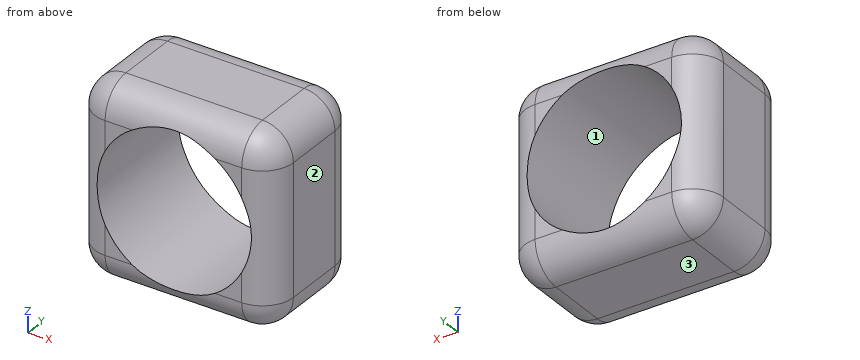
Autodesk Inventor part; units mm, degrees
ref_plane "YZ Plane" through (0, 0, 0) normal (1, 0, 0) x (0, 1, 0)
ref_plane "XZ Plane" through (0, 0, 0) normal (0, 1, 0) x (-1, 0, 0)
ref_plane "XY Plane" through (0, 0, 0) normal (0, 0, 1) x (1, 0, 0)
sketch "Sketch1" plane through (0, 0, 0) normal (0, 1, 0) x (-1, 0, 0)
  circle A0 centre (0, 0) radius 5
  line L0 (6.4276, 6.2219) -> (-6.4276, 6.2219)
  line L1 (-6.4276, 6.2219) -> (-6.4276, -6.2219)
  line L2 (-6.4276, -6.2219) -> (6.4276, -6.2219)
  line L3 (6.4276, -6.2219) -> (6.4276, 6.2219)
  line L4 (6.4276, 6.2219) -> (-6.4276, -6.2219) construction
  line L5 (-6.4276, 6.2219) -> (6.4276, -6.2219) construction
  dimension "d0" = 10
extrude "Extrusion1" add sketch "Sketch1" along normal blind 8
fillet "Fillet1" radius 2 12 edges at (6.4276, 8, 0) (0, 8, -6.2219) (0, 8, 6.2219) (-6.4276, 8, 0) (-6.4276, 0, 0) (0, 0, 6.2219) (6.4276, 0, 0) (0, 0, -6.2219) (-6.4276, 4, -6.2219) (6.4276, 4, 6.2219) (6.4276, 4, -6.2219) (-6.4276, 4, 6.2219)
thread "Thread1"
properties part number "benzcadnut"
The model under review builds one solid part; all positions refer to its coordinate system, in mm. Face numbers are marked on the shaded views. Round coordinates to 2 decimals unless told otherwise and drop trailing zeros. Order: outer loops, then holes, each group sorted by start corner. A loop starts at its lowest first (then second) coordinate and runs counter-clockwise, first axis right, second up.
Item 1: Add section D-D, the plane z = 0.75. State the section outline as (x, y) points, and give its area (3 significant figures).
Working result:
outline: (-6.43, 2) arc R2 ccw to (-4.94, 0.07) - (-4.94, 7.93) arc R2 ccw to (-6.43, 6) - close; (4.94, 0.07) arc R2 ccw to (6.43, 2) - (6.43, 6) arc R2 ccw to (4.94, 7.93) - close
area: 20.4 mm2
Item 2: To check wall thickness, follow probe 1 along X at (y, z) = (3.25, 0); probe 2 along Z at (x, y) = (0, 5.5); probe 3 along Z at (x, y) = (3, 5). State the ranges of each line that lie inside material, in increasing order.
Working result:
probe 1: x = -6.43 to -5, 5 to 6.43
probe 2: z = -6.22 to -5, 5 to 6.22
probe 3: z = -6.22 to -4, 4 to 6.22
Item 3: Draft analysis for pull direction Z (two halves, no side actions). For the marked faces 1, 2 and 3, state which applies: released by +Z, released by -Z, zero draft, split by the parting line, or undercut.
Working result:
face 1: undercut
face 2: zero draft
face 3: released by -Z
Item 4: Add section A-A, the plane x = -4. State the section outline as (y, z) points.
Working result:
outline: (0, -4.22) arc R2 ccw to (2, -6.22) - (6, -6.22) arc R2 ccw to (8, -4.22) - (8, -3) - (0, -3) - close; (0, 3) - (8, 3) - (8, 4.22) arc R2 ccw to (6, 6.22) - (2, 6.22) arc R2 ccw to (0, 4.22) - close
Item 5: Add section B-B, the plane y = 3.5. State the section outline as (x, z) points.
Working result:
outline: (-6.43, -4.22) arc R2 ccw to (-4.43, -6.22) - (4.43, -6.22) arc R2 ccw to (6.43, -4.22) - (6.43, 4.22) arc R2 ccw to (4.43, 6.22) - (-4.43, 6.22) arc R2 ccw to (-6.43, 4.22) - close; hole circle Ø10 at (0, 0)
Item 6: Add section C-C, the plane z = -3.75. State the section outline as (x, y) points, and give its area (3 significant figures).
Working result:
outline: (-6.43, 2) arc R2 ccw to (-4.43, 0) - (-3.31, 0) - (-3.31, 8) - (-4.43, 8) arc R2 ccw to (-6.43, 6) - close; (3.31, 0) - (4.43, 0) arc R2 ccw to (6.43, 2) - (6.43, 6) arc R2 ccw to (4.43, 8) - (3.31, 8) - close
area: 46.5 mm2
